Autodesk Inventor part; units mm, degrees
ref_plane "YZ Plane" through (0, 0, 0) normal (1, 0, 0) x (0, 1, 0)
ref_plane "XZ Plane" through (0, 0, 0) normal (0, 1, 0) x (-1, 0, 0)
ref_plane "XY Plane" through (0, 0, 0) normal (0, 0, 1) x (1, 0, 0)
sketch "Boceto1" plane through (0, 0, 0) normal (0, 1, 0) x (-1, 0, 0)
  line L0 (0, 0) -> (-102, 0)
  line L1 (-102, 0) -> (-102, -16.2)
  line L2 (-96, -22.2) -> (-6, -22.2)
  line L3 (0, -16.2) -> (0, 0)
  arc A0 (-102, -16.2) -> (-96, -22.2) centre (-96, -16.2) ccw
  arc A1 (-6, -22.2) -> (0, -16.2) centre (-6, -16.2) ccw
  line L4 (0, 0) -> (-51, 0) construction
  line L5 (-51, 0) -> (-51, -11.1) construction
  circle A2 centre (-6, -16.2) radius 4
  circle A3 centre (-96, -16.2) radius 4
  dimension "d0" = 6
  dimension "d1" = 102
  dimension "d2" = 22.2
  dimension "d3" = 51
  dimension "d4" = 11.1
  dimension "d5" = 8
  dimension "d6" = 8
extrude "Extrusión1" add sketch "Boceto1" along normal blind 22.2 contours L3 A1 L2 A0 L1 L0 | A2 | A3
sketch "Boceto2" plane through (0, 22.2, 0) normal (0, 1, 0) x (1, 0, 0)
  arc A0 (6, 22.2) -> (0, 16.2) centre (6, 16.2) ccw
  circle A1 centre (6, 16.2) radius 4
  arc A2 (102, 16.2) -> (96, 22.2) centre (96, 16.2) ccw
  circle A3 centre (96, 16.2) radius 4
  point P0 (0, 0)
  dimension "d9" = 8
  dimension "d10" = 8
extrude "Extrusión2" cut sketch "Boceto2" against normal through all
sketch "Boceto3" plane through (96, 0, -22.2) normal (0, 0, -1) x (-1, 0, 0)
  line L0 (-6, 0) -> (-6, 22.2)
  line L1 (96, 0) -> (96, 22.2)
  line L2 (0, 0) -> (90, 0)
  line L3 (0, 22.2) -> (90, 22.2)
  line L4 (96, 22.2) -> (90, 22.2)
  line L5 (96, 0) -> (90, 0)
  line L6 (0, 0) -> (-6, 0)
  line L7 (0, 22.2) -> (-6, 22.2)
  line L8 (-6, 0) -> (45, 0) construction
  line L9 (45, 0) -> (45, 11.1) construction
  arc A0 (69.44, 15.35) -> (69.44, 6.85) centre (69.44, 11.1) ccw
  line L10 (69.44, 6.85) -> (96, 6.85)
  line L11 (96, 15.35) -> (69.44, 15.35)
  arc A1 (20.56, 6.85) -> (20.56, 15.35) centre (20.56, 11.1) ccw
  line L12 (20.56, 6.85) -> (-6, 6.85)
  line L13 (-6, 15.35) -> (20.56, 15.35)
  circle A2 centre (45, 11.1) radius 6.25
  dimension "d13" = 51
  dimension "d14" = 11.1
  dimension "d15" = 8.5
  dimension "d16" = 26.56
  dimension "d17" = 12.5
extrude "Extrusión3" cut sketch "Boceto3" against normal through all contours L0 L13 A1 L12 | L10 A0 L11 L1 | A2
equation "\"Radio_pliegue\" = Grosor"
equation "\"Anchura_desahogo_plegado\" = Grosor"
equation "\"Profundidad_desahogo_plegado\" = 0.5 * Grosor"
equation "\"Tamaño_destalonado\" = 4 * Grosor"
equation "\"Remanente_mínimo\" = 2 * Grosor"
equation "\"Radiodetransición\" = Radio_pliegue"
equation "\"Tamaño_de_radio_de_Jacobi\" = Radio_pliegue"
equation "\"TamañoSeparación\" = Grosor"
properties part number "Practica 7" material "Hierro, gris"
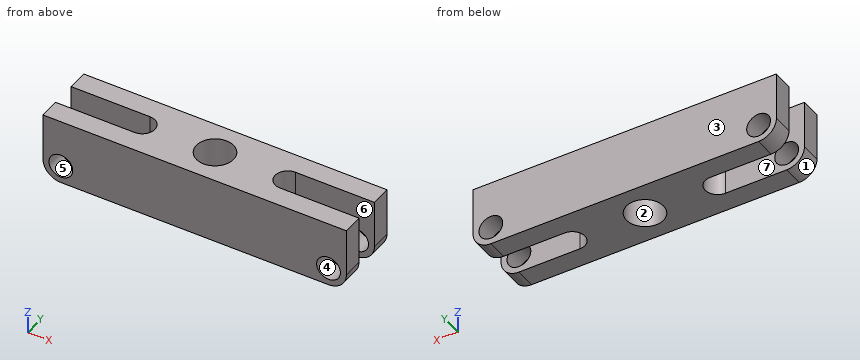
Build history of the part. All positions in model axes, mm. Face numbers are marked on the shaded views. A direction names the side the tool comes from. Give positions to 0.01 mm unless a question says otherwise; leave off trailing zeros. Order: outer loops, then holes, each group sorted by start corner. A loop starts at its lowest first (then second) coordinate and runs counter-clockwise, first axis right, second up. Notation, with made-up numbers: M 45,43.5 L 62,43.5 A31 cw 62,80.5 Z; hole C 86.5,-2.75 d6. An arc over 180 degrees is marked long. Write item = value, one per line. Start each with the question number.
(1) Slice it at A-A on x = 78. Write the cut outline in (y, z), plus the area to 3 significant figures.
(2) Which spindle directions (+Z, -Z, +X, -X, +Y, -Y) get a long thin tool onto all of the face, cutting with end or side? Do the marked faces 5, 6 and 7. Say none if no direction does.
(3) Probe L1, parallel to X at y = 19, z = -16.2; L2, parallel to Y at x = 77.5, z = -10.5; L3, parallel to Y at x = 51, z = -14.5. List the from-to ranges inside material, lowest first. Write a range as [from, to].
(4) Slice it at B-B on z = -9.5. Write the cut outline in (x, y).
(5) Slice it at D-D on z = -18.75. State how many separate pieces and enclosed holes the cut face has, plus the area to 3 significant figures.
(6) Two-plate mould, pull along X, no slides. Class the marked faces 1, 2, 3 and 4: released by +X, released by -X, zero draft, split by the parting line, or undercut.
(7) Slice it at C-C on y = 11.1. Write the cut outline in (x, z).
(8) Pin check, flat tips, straight feed: pin 1 Ø1 at (y, z) = (10.5, -3) entering from +X; pin 2 Ø3 at (y, z) = (12.5, -4.5) entering from +X. Stop position of each tip, or through.
Responses:
q1.outline = M 0,-22.2 L 6.85,-22.2 L 6.85,0 L 0,0 Z; M 15.35,-22.2 L 22.2,-22.2 L 22.2,0 L 15.35,0 Z
q1.area = 304 mm2
q2.face_5 = +Y, -Y
q2.face_6 = +Z, -Z, +X
q2.face_7 = +Z, -Z, -X
q3.L1 = [0, 2], [10, 92], [100, 102]
q3.L2 = [0, 6.85], [15.35, 22.2]
q3.L3 = [0, 4.85], [17.35, 22.2]
q4.outline = M 0,0 L 102,0 L 102,6.85 L 75.44,6.85 A4.25 cw 75.44,15.35 L 102,15.35 L 102,22.2 L 0,22.2 L 0,15.35 L 26.56,15.35 A4.25 cw 26.56,6.85 L 0,6.85 Z; hole C 51,11.1 d12.5
q5.separate_pieces = 5
q5.enclosed_holes = 1
q5.area = 1,450 mm2
q6.face_1 = released by -X
q6.face_2 = undercut
q6.face_3 = zero draft
q6.face_4 = undercut
q7.outline = M 30.81,-22.2 L 44.75,-22.2 L 44.75,0 L 30.81,0 Z; M 57.25,-22.2 L 71.19,-22.2 L 71.19,0 L 57.25,0 Z
q8.pin_1 = 71.33
q8.pin_2 = 72.33
